Can you work these out from the model? Positions are in its coordinate system, mm. Face numbers are marked on the shaded views. Round coordinates to 2 decimals unless told otherwise and drop trailing zeros. Write each loop counter-clockwise with the first axis right and the second up, starting at its lowest first coordinate (ties: lowest second). Pieces come first, ordered by that corner, then holes.
Q1. We'd pull the mould along Y, two halves only. Please class the marked faces 1 and 2: +Y half, -Y half, draft (parallel to the pull), parting line (faces both ways), or undercut.
Q2. If we section it at B-B (x = -4.25): Please give me the cut outline in (y, z).
Q3. Please list where these lines run through material, in increasing order: line 1 along Y through (x, z) = (0.5, 40.5); line 2 along X through (y, z) = (1.75, 57); line 3 along Y through (x, z) = (-7.75, 30).
Q4. If we section it at C-C (x = 9.75): Please give me the cut outline in (y, z), plus the area to 3 significant figures.
Q5. If we section it at A-A (y = -2.25): Please give me the cut outline in (x, z).
Q6. I'm going to push flat-ended pins straight in: pin 1 Ø2 at (y, z) = (6.5, 34.5) entering from +X; pin 2 Ø5 at (y, z) = (1, 50.5) entering from -X; pin 3 Ø6 at (y, z) = (6, 31) entering from +X; pin 4 Ø0.7 at (y, z) = (9, 60) entering from -X. Where does each tip first touch, or does it pass through?
Q7. If we section it at D-D (z = 24): Please give me the cut outline in (x, y).
from build123d import *

# Parameters (mm, degrees)
F0_R          = 11.25
F0_R_2        = 10.5
F1_DEPTH      = 76.2
F2_W          = 11.43
F2_H          = 20.6375
F3_DEPTH      = 25.4
F5_DEPTH      = 25.4
F5_DEPTH_BACK = 25.4


with BuildPart() as f1:
    # F0 (on Top) → F1 (new body)
    with BuildSketch(Plane.XY):
        Circle(F0_R)
        Circle(F0_R_2, mode=Mode.SUBTRACT)
    extrude(amount=F1_DEPTH)

    # F2 (on Front) → F3 (cut)
    with BuildSketch(Plane.XZ):
        with Locations((0, 61.11875)):
            Rectangle(F2_W, F2_H)
    extrude(amount=-F3_DEPTH, mode=Mode.SUBTRACT)

    # F4 (on Front) → F5 (cut, two sides)
    with BuildSketch(Plane.XZ) as f5_sk:
        with BuildLine():
            ThreePointArc((0, 2.7625), (1.4142135624, 3.3482864376), (2, 4.7625))
            ThreePointArc((2, 4.7625), (-1.4142135624, 6.1767135624), (0, 2.7625))
        make_face()
    extrude(amount=-F5_DEPTH, mode=Mode.SUBTRACT)
    extrude(f5_sk.sketch, amount=F5_DEPTH_BACK, mode=Mode.SUBTRACT)


solid = f1.part
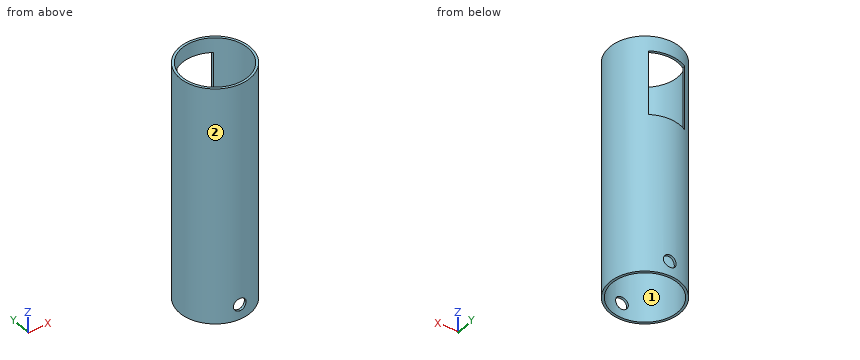
A:
1. face 1: undercut
1. face 2: parting line
2. outline: (-10.42, 0) - (-9.6, 0) - (-9.6, 76.2) - (-10.42, 76.2) - close; (9.6, 0) - (10.42, 0) - (10.42, 50.8) - (9.6, 50.8) - close; (9.6, 71.44) - (10.42, 71.44) - (10.42, 76.2) - (9.6, 76.2) - close
3. line 1: y = -11.24 to -10.49, 10.49 to 11.24
3. line 2: x = -11.11 to -10.35, 10.35 to 11.11
3. line 3: y = -8.15 to -7.08, 7.08 to 8.15
4. outline: (-5.61, 0) - (-3.9, 0) - (-3.9, 76.2) - (-5.61, 76.2) - close; (3.9, 0) - (5.61, 0) - (5.61, 76.2) - (3.9, 76.2) - close
4. area: 261 mm2
5. outline: (-11.02, 0) - (-10.26, 0) - (-10.26, 76.2) - (-11.02, 76.2) - close; (10.26, 0) - (11.02, 0) - (11.02, 76.2) - (10.26, 76.2) - close
6. pin 1: stops at x = 9.81
6. pin 2: stops at x = -11.25
6. pin 3: stops at x = 10.84
6. pin 4: stops at x = -7.19
7. outline: circle Ø22.5 at (0, 0); hole circle Ø21 at (0, 0)
